For this review, take the finished solid that the model builds, in its own axes (mm). A direction names the side the tool comes from. Round coordinates to 2 decimals unless told otherwise and drop trailing zeros. Loops run counter-clockwise (first coordinate to the right, second up) from the corner with the lowest first, then second, coordinate; pieces in that order, holes last. Notation, with made-up numbers: (-3.75, 61) -> (34.25, 61) arc R21 ccw to (34.25, 76) -> close; hole circle Ø1 at (-6, -27). An arc over 180 degrees is marked (long way). Write each question's results on one line, items separated by ' | '.
```python
from build123d import *

# Parameters (mm, degrees)
EXTRUDE_3_DEPTH     = 10
CUT_EXTRUDE_2_DEPTH = 8
CUT_EXTRUDE_4_DEPTH = 8
CUT_EXTRUDE_5_DEPTH = 8


with BuildPart() as part:
    # 草图1 → 凸台-拉伸3 (new body)
    with BuildSketch(Plane.XY):
        Polygon((0, 0), (35, 0), (35, 35), (33.594225436, 35), (0, 1), align=None)
    extrude(amount=EXTRUDE_3_DEPTH)

    # 草图4 → 切除-拉伸2 (cut)
    with BuildSketch(Plane.XY.offset(10)):
        Polygon((3.799665242, 2), (33, 2), (33, 31.553036836), (33, 35.783784072), (-1.057608141, 2), align=None)
    extrude(amount=-CUT_EXTRUDE_2_DEPTH, mode=Mode.SUBTRACT)

    # 草图7 → 切除-拉伸4 (cut)
    with BuildSketch(Plane(origin=(0, 2, 0), x_dir=(1, 0, 0), z_dir=(0, 1, 0))):
        with BuildLine():
            Line((7.669292291, -8), (27.669292291, -8))
            ThreePointArc((27.669292291, -8), (29.669292291, -10), (27.669292291, -12))
            Line((27.669292291, -12), (7.669292291, -12))
            ThreePointArc((7.669292291, -12), (5.669292291, -10), (7.669292291, -8))
        make_face()
    extrude(amount=-CUT_EXTRUDE_4_DEPTH, mode=Mode.SUBTRACT)

    # 草图8 → 切除-拉伸5 (cut)
    with BuildSketch(Plane.ZY.offset(-33)):
        with BuildLine():
            Line((12, 28.042571575), (12, 8.042571575))
            ThreePointArc((12, 8.042571575), (10, 6.042571575), (8, 8.042571575))
            Line((8, 8.042571575), (8, 28.042571575))
            ThreePointArc((8, 28.042571575), (10, 30.042571575), (12, 28.042571575))
        make_face()
    extrude(amount=-CUT_EXTRUDE_5_DEPTH, mode=Mode.SUBTRACT)

    # 镜向3: part across plane


with BuildPart() as part_1:
    add(part.part)
    add(part.part.mirror(Plane(origin=(0, 35, 10), x_dir=(1, 0, 0), z_dir=(0, 0, 1))))


solid = part_1.part
```
1. To check wall thickness, follow probe 1 along Z at (x, y) = (14, 9); probe 2 along Z at (x, y) = (33.5, 24.5); probe 3 along X at (y, z) = (19, 13). State the ranges of each line that lie inside material, in increasing order.
Values found:
probe 1: z = 0 to 2, 18 to 20 | probe 2: z = 0 to 8, 12 to 20 | probe 3: x = 33 to 35
2. Consider section B-B (z = 14.5). State the section outline as (x, y) points.
Values found:
outline: (0, 0) -> (35, 0) -> (35, 35) -> (33.59, 35) -> (33, 34.4) -> (33, 2) -> (0.99, 2) -> (0, 1) -> close
3. Tool access review of faces 1 (the face through (17.3, 0, 12.4)), 2 (the face through (33.986, 6.043, 9.956)), 3 (the face through (5.67, 1.01, 9.96)), 4 (the face through (24, 11, 18)): name each direction out of +Z, -Z, +X, -X, +Y, -Y from which nothing blocks a thin tool from reaching the whole face with its end or side.
Values found:
face 1: +Z, -Z, +X, -X, -Y | face 2: +X, -X | face 3: +Y, -Y | face 4: -X, +Y
4. Draft analysis for pull direction Z (two halves, no side actions). For faces 5 (the face through (29.67, 1.01, 10.04)), 6 (the face through (16.875, 18.079, 18.195)), 7 (the face through (21, 14, 0)), state which applies: released by +Z, released by -Z, zero draft, split by the parting line, or undercut.
Values found:
face 5: undercut | face 6: zero draft | face 7: released by -Z
5. For pin 1 (1 mm diameter, centred on x = 17, z = 12, fed in from +Y); pin 2 (8 mm diameter, centred on y = 16.5, z = 10, fed in from -X), all flat-tipped, find the tip position at first contact; note any pin that passes through.
Values found:
pin 1: stops at y = 2 | pin 2: stops at x = 33
6. Consider section A-A (z = 10). State the section outline as (x, y) points.
Values found:
outline: (0, 0) -> (5.67, 0) -> (5.67, 2) -> (0.99, 2) -> (0, 1) -> close; (29.67, 0) -> (35, 0) -> (35, 6.04) -> (33, 6.04) -> (33, 2) -> (29.67, 2) -> close; (33, 30.04) -> (35, 30.04) -> (35, 35) -> (33.59, 35) -> (33, 34.4) -> close
7. Consider section C-C (x = 19). State the section outline as (y, z) points.
Values found:
outline: (0, 0) -> (20.23, 0) -> (20.23, 2) -> (2, 2) -> (2, 8) -> (0, 8) -> close; (0, 12) -> (2, 12) -> (2, 18) -> (20.23, 18) -> (20.23, 20) -> (0, 20) -> close
8. Consider section D-D (y = 18). State the section outline as (x, z) points.
Values found:
outline: (16.8, 0) -> (35, 0) -> (35, 8) -> (33, 8) -> (33, 2) -> (16.8, 2) -> close; (16.8, 18) -> (33, 18) -> (33, 12) -> (35, 12) -> (35, 20) -> (16.8, 20) -> close
